Can you work these out from the model? Positions are in its coordinate system, mm. Round coordinates to 2 decimals unless told otherwise and drop trailing zeros. Loops run counter-clockwise (first coordinate to the right, second up) from the corner with the lowest first, then second, coordinate; pieces in that order, holes last.
Autodesk Inventor part; units mm, degrees
ref_plane "XZ Plane" through (0, 0, 0) normal (0, 1, 0) x (-1, 0, 0)
ref_plane "XY Plane" through (0, 0, 0) normal (0, 0, 1) x (1, 0, 0)
sketch "Sketch1" plane through (0, 0, 0) normal (0, 1, 0) x (-1, 0, 0)
  line L0 (0, 0) -> (-180, 0)
  line L1 (-180, 0) -> (-180, 20)
  line L2 (-180, 20) -> (0, 20)
  line L3 (0, 20) -> (0, 0)
  dimension "d0" = 180
  dimension "d1" = 20
extrude "Extrusion1" add sketch "Sketch1" along normal blind 2
hole "Hole1" at (8, 2, 10.2209) direction (0, -1, 0) diameter 5.5 end through all
pattern_linear "Rectangular Pattern1" count 2 spacing 166 along (1, 0, 0) of "Hole1"
sketch "Sketch2" plane through (0, 2, 0) normal (0, 1, 0) x (1, 0, 0)
  line L0 (0, -20) -> (180, -20)
  line L1 (90, -20) -> (90, 0) construction
  line L2 (90, -10) -> (115, -10) construction
  point P0 (0, 0)
  dimension "d16" = 25
hole "Hole2" at (115, 2, 10) direction (0, -1, 0) diameter 5.5 end through all
ref_plane "Work Plane1" through (90, 0, 0) normal (1, 0, 0) x (0, 1, 0)
mirror "Mirror1" about plane through (90, 0, 0) normal (1, 0, 0) of "Hole2"
properties part number "flat bar1" material "Aluminum 6061"
(1) If we section it at A-A, the plane x = 65: List the corners of the cut face in (y, z) for me, then the cut area to 3 significant figures.
Worked answers:
outline: (0, 0) - (2, 0) - (2, 7.25) - (0, 7.25) - close; (0, 12.75) - (2, 12.75) - (2, 20) - (0, 20) - close
area: 29.0 mm2
(2) Will this pin go through, and if not, where does the flat tip stop? P1, Ø4.5, axis at x = 8, z = 10.22, coming from the +Y side.
Worked answers:
P1: passes through
(3) If we section it at C-C, the plane z = 10: List the corners of the cut face in (x, y) for me.
Worked answers:
outline: (0, 0) - (5.26, 0) - (5.26, 2) - (0, 2) - close; (10.74, 0) - (62.25, 0) - (62.25, 2) - (10.74, 2) - close; (67.75, 0) - (112.25, 0) - (112.25, 2) - (67.75, 2) - close; (117.75, 0) - (171.26, 0) - (171.26, 2) - (117.75, 2) - close; (176.74, 0) - (180, 0) - (180, 2) - (176.74, 2) - close
(4) If I drill on line 1 (X direction, y = 1.35, z = 10); line 2 (X direction, y = 1, z = 8.75); line 3 (Z direction, x = 8, y = 0.8), over which ranges is the centre line in solid material (lowest first)?
Worked answers:
line 1: x = 0 to 5.26, 10.74 to 62.25, 67.75 to 112.25, 117.75 to 171.26, 176.74 to 180
line 2: x = 0 to 5.68, 10.32 to 62.55, 67.45 to 112.55, 117.45 to 171.68, 176.32 to 180
line 3: z = 0 to 7.47, 12.97 to 20
(5) If we mould it in two halves opening along Z, with no side actions, what happens to faces 1 (the flat face through (91, 2, 10)), 2 (the cylindrical face through (62.273, 0.986, 9.642))? For each: released by +Z, released by -Z, zero draft, split by the parting line, or undercut.
Worked answers:
face 1: zero draft
face 2: undercut
(6) If we section it at B-B, the plane y = 0.65: List the corners of the cut face in (x, z) for me, then the cut area to 3 significant figures.
Worked answers:
outline: (0, 0) - (180, 0) - (180, 20) - (0, 20) - close; hole circle Ø5.5 at (8, 10.22); hole circle Ø5.5 at (65, 10); hole circle Ø5.5 at (115, 10); hole circle Ø5.5 at (174, 10.22)
area: 3,500 mm2
